Verification items for the finished model (mm, model axes). Face numbers are marked on the shaded views. Round coordinates to 2 decimals unless told otherwise and drop trailing zeros. Loops run counter-clockwise (first coordinate to the right, second up) from the corner with the lowest first, then second, coordinate; pieces in that order, holes last. Notation, with made-up numbers: M 86,67.5 L 132,67.5 A19 cw 132,96.5 Z; hole C -39.5,8.5 d11. An arc over 180 degrees is marked long. Answer as CSV lines item,"result".
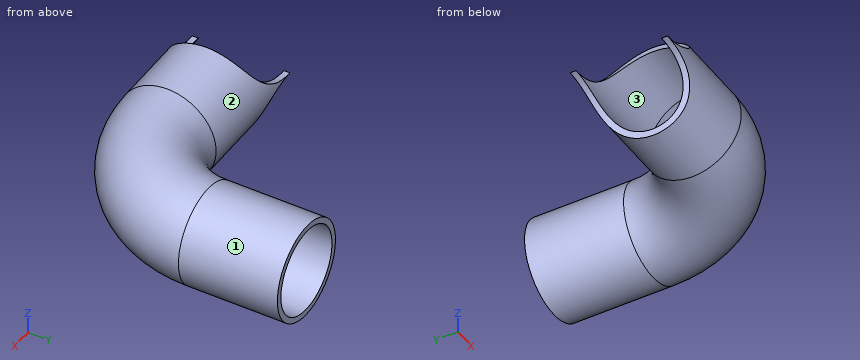
```python
from build123d import *

# Parameters (mm, degrees)
SKETCH1_R          = 12.5
SKETCH3_R          = 11
SKETCH7_R          = 15.157577
CUT_EXTRUDE1_DEPTH = 81.367795269


with BuildPart() as part:
    # Sweep1: sweep along a path in Sketch2
    with BuildLine(Plane.XY) as sweep1_path:
        Line((0, 0), (31.75, 0))
        ThreePointArc((31.75, 0), (49.710512242, 7.439487758), (57.15, 25.4))
        Line((57.15, 25.4), (57.15, 50.8))
    # Sketch1 → Sweep1 (sweep)
    with BuildSketch(Plane(origin=(0, 0, 0), x_dir=(0, 0, -1), z_dir=(1, 0, 0))):
        Circle(SKETCH1_R)
    sweep(path=sweep1_path.line)

    # Cut-Sweep1: sweep along a path in Sketch2<2>
    with BuildLine(Plane.XY) as cut_sweep1_path:
        Line((0, 0), (31.75, 0))
        ThreePointArc((31.75, 0), (49.710512242, 7.439487758), (57.15, 25.4))
        Line((57.15, 25.4), (57.15, 50.8))
    # Sketch3 → Cut-Sweep1 (sweep, cut)
    with BuildSketch(Plane.ZY):
        Circle(SKETCH3_R)
    sweep(path=cut_sweep1_path.line, mode=Mode.SUBTRACT)

    # Sketch7 → Cut-Extrude1 (cut, through all)
    with BuildSketch(Plane(origin=(0, 12.7, 0), x_dir=(1, 0, 0), z_dir=(0, 1, 0))):
        with Locations((0, 15.157577)):
            Circle(SKETCH7_R)
    cut_extrude1 = extrude(amount=-CUT_EXTRUDE1_DEPTH, mode=Mode.SUBTRACT)

    # Mirror1: Cut-Extrude1 across plane
    add(cut_extrude1.mirror(Plane.XY), mode=Mode.SUBTRACT)


solid = part.part
```
1) Section check B-B (y = 40). Record the cut outline in (x, z).
Here are the results:
outline,"C 57.15,0 d25; hole C 57.15,0 d22"
2) Go/stop test with flat-tipped pins: pin 1 (4 mm diameter, centred on x = 29, y = 12, fed in from -Z); pin 2 (10 mm diameter, centred on x = 56, z = -8.5, fed in from -Y); pin 3 (10 mm diameter, centred on x = 58, z = -4.5, fed in from -Y). Record where each tip stops, or that it passes through.
Here are the results:
pin 1,"stops at z = -7.5"
pin 2,"stops at y = -5.13"
pin 3,"stops at y = -5.39"
3) Section check D-D (z = 3). Record the cut outline in (x, y).
Here are the results:
outline,"M 9.05,-12.13 L 31.75,-12.13 A37.53 ccw 69.28,25.4 L 69.28,50.8 L 67.73,50.8 L 67.73,25.4 A35.98 cw 31.75,-10.58 L 9.05,-10.58 Z; M 9.05,10.58 L 31.75,10.58 A14.82 ccw 46.57,25.4 L 46.57,50.8 L 45.02,50.8 L 45.02,25.4 A13.27 cw 31.75,12.13 L 9.05,12.13 Z"
4) Section check A-A (z = -6.75). Record the cut outline in (x, y), plus the area to 3 significant figures.
Here are the results:
outline,"M 12.61,-10.52 L 31.75,-10.52 A35.92 ccw 67.67,25.4 L 67.67,50.8 L 65.84,50.8 L 65.84,25.4 A34.09 cw 31.75,-8.69 L 12.61,-8.69 Z; M 12.61,8.69 L 31.75,8.69 A16.71 ccw 48.46,25.4 L 48.46,50.8 L 46.63,50.8 L 46.63,25.4 A14.88 cw 31.75,10.52 L 12.61,10.52 Z"
area,"310 mm^2"
5) Material ranges on probe 1 along X at (y, z) = (45, 0); probe 2 along Y at (x, z) = (13, 0), recorded low to high.
Here are the results:
probe 1,"x = 44.65 to 46.15, 68.15 to 69.65"
probe 2,"y = -12.5 to -11, 11 to 12.5"
6) Draft check along Y on the marked faces 1, 2 and 3. Enter one of: +Y half, -Y half, draft (parallel to the pull), parting line (faces both ways), or undercut.
Here are the results:
face 1,"draft"
face 2,"parting line"
face 3,"undercut"
7) Section check C-C (x = 28.5). Record the cut outline in (y, z).
Here are the results:
outline,"C 0,0 d25; hole C 0,0 d22"
